Source: CAD feature listing. Evaluate the final solid. Frame: model axes, mm. A direction names the side the tool comes from. Give positions to 0.01 mm unless a question says otherwise; leave off trailing zeros. Order: outer loops, then holes, each group sorted by start corner. A loop starts at its lowest first (then second) coordinate and runs counter-clockwise, first axis right, second up. Notation, with made-up numbers: (68, -28) - (120, -28) arc R23 cw to (120, -15) - close; hole circle Ø7 at (74, 89). An arc over 180 degrees is marked (long way). Write each question's results on one line, items separated by ' | '. Start each with the question number.
Item 1: Line query: line 1 along Y through (x, z) = (9, -4.5); line 2 along X through (y, z) = (-5, -1). Output: solid intervals per line, ascending.
Item 2: Section C-C on y = 8. Output: boundary loops of the cut face in (x, z).
Item 3: Set-up query: faces 1 (the cylindrical face through (-16.129, 16.254, 5.059)), 2 (the flat face through (21, -10.5, -14)), 3 (the conical face through (16.37, 16.24, 3.74)). Return all of +Z, -Z, +X, -X, +Y, -Y with unobstructed straight access to the full face (end or side cutting, diameter ignored); none if empty.
Item 4: Mould query, pull axis Y, two halves, no side actions, for faces 4 (the cylindrical face through (-18.192, 18.363, -12.977)), 5 (the flat face through (-19, 0, 6.25)), 6 (the cylindrical face through (20.514, -9.297, -1.891)). Classes: released by +Y, released by -Y, zero draft, split by the parting line, or undercut.
Item 5: Section B-B on z = -8.5. Output: boundary loops of the cut face in (x, y), and give its area (3 significant figures).
Item 6: Contact query for flat-ended pins moving along their axis: pin 1 Ø1 at (x, z) = (21, -18) entering from +Y; pin 2 Ø2 at (x, z) = (-16, -10) entering from -Y; pin 3 Ø1.6 at (x, z) = (20, -12) entering from -Y. Output: stop coordinate, or through.
Item 7: Section A-A on x = -3. Output: boundary loops of the cut face in (y, z), and give its area (3 significant figures).
Item 8: Section D-D on y = -9.5. Output: boundary loops of the cut face in (x, z), and give its area (3 significant figures).
```python
from build123d import *

# Parameters (mm, degrees)
POWER_BUTTON_HOLE_DEPTH = 2


with BuildPart() as part:
    # Case 2: sweep along a path in Sketch1
    with BuildLine(Plane.XY) as case_2_path:
        Line((-10.5, -19.25), (10.5, -19.25))
        ThreePointArc((10.5, -19.25), (16.687184335, -16.687184335), (19.25, -10.5))
        Line((19.25, -10.5), (19.25, 10.5))
        ThreePointArc((19.25, 10.5), (16.687184335, 16.687184335), (10.5, 19.25))
        Line((10.5, 19.25), (-10.5, 19.25))
        ThreePointArc((-10.5, 19.25), (-16.687184335, 16.687184335), (-19.25, 10.5))
        Line((-19.25, 10.5), (-19.25, -10.5))
        ThreePointArc((-19.25, -10.5), (-16.687184335, -16.687184335), (-10.5, -19.25))
    # Sketch4 → Case 2 (sweep)
    with BuildSketch(Plane(origin=(0, 0, 0), x_dir=(1, 0, 0), z_dir=(0, 1, 0))):
        with BuildLine():
            Line((-19.5, 0), (-19.5, -3))
            Line((-19.5, -3), (-19.45, -3))
            Line((-19.45, -3), (-18.55, -3.9))
            Line((-18.55, -3.9), (-18.55, -6.25))
            Line((-18.55, -6.25), (-21.5, -6.25))
            Line((-21.5, -6.25), (-21.5, 32.75))
            Line((-21.5, 32.75), (-19.5, 32.75))
            Line((-19.5, 32.75), (-19.5, 31.616025404))
            ThreePointArc((-19.5, 31.616025404), (-19.566987298, 31.366025404), (-19.75, 31.183012702))
            ThreePointArc((-19.75, 31.183012702), (-20, 30.75), (-19.75, 30.316987298))
            ThreePointArc((-19.75, 30.316987298), (-19.566987298, 30.133974596), (-19.5, 29.883974596))
            Line((-19.5, 29.883974596), (-19.5, 0))
        make_face()
    sweep(path=case_2_path.line)

    # Sketch6 → Power Button Hole (cut)
    with BuildSketch(Plane(origin=(21.5, 0, 0), x_dir=(0, 0, -1), z_dir=(1, 0, 0))):
        with BuildLine():
            Line((23.75, 10.5), (4.75, 10.5))
            ThreePointArc((4.75, 10.5), (1.921572875, 9.328427125), (0.75, 6.5))
            Line((0.75, 6.5), (0.75, -6.5))
            ThreePointArc((0.75, -6.5), (1.921572875, -9.328427125), (4.75, -10.5))
            Line((4.75, -10.5), (23.75, -10.5))
            ThreePointArc((23.75, -10.5), (26.578427125, -9.328427125), (27.75, -6.5))
            Line((27.75, -6.5), (27.75, 6.5))
            ThreePointArc((27.75, 6.5), (26.578427125, 9.328427125), (23.75, 10.5))
        make_face()
    extrude(amount=-POWER_BUTTON_HOLE_DEPTH, mode=Mode.SUBTRACT)


solid = part.part
```
Evaluation:
1) line 1: y = -21.5 to -19.5, 19.5 to 21.5 | line 2: x = -21.5 to -19.5
2) outline: (-21.5, -32.75) - (-19.5, -32.75) - (-19.5, -31.62) arc R0.5 ccw to (-19.75, -31.18) arc R0.5 cw to (-19.75, -30.32) arc R0.5 ccw to (-19.5, -29.88) - (-19.5, 3) - (-19.45, 3) - (-18.55, 3.9) - (-18.55, 6.25) - (-21.5, 6.25) - close; (18.55, 3.9) - (19.45, 3) - (19.5, 3) - (19.5, -1.04) - (21.5, -1.04) - (21.5, 6.25) - (18.55, 6.25) - close; (19.5, -32.75) - (21.5, -32.75) - (21.5, -27.46) - (19.5, -27.46) - (19.5, -29.88) arc R0.5 ccw to (19.75, -30.32) arc R0.5 cw to (19.75, -31.18) arc R0.5 ccw to (19.5, -31.62) - close
3) face 1: +Z, -Z | face 2: +X | face 3: -Z
4) face 4: released by +Y | face 5: zero draft | face 6: undercut
5) outline: (-21.5, -10.5) arc R11 ccw to (-10.5, -21.5) - (10.5, -21.5) arc R11 ccw to (21.5, -10.5) - (19.5, -10.5) arc R9 cw to (10.5, -19.5) - (-10.5, -19.5) arc R9 cw to (-19.5, -10.5) - (-19.5, 10.5) arc R9 cw to (-10.5, 19.5) - (10.5, 19.5) arc R9 cw to (19.5, 10.5) - (21.5, 10.5) arc R11 ccw to (10.5, 21.5) - (-10.5, 21.5) arc R11 ccw to (-21.5, 10.5) - close | area: 252 mm^2
6) pin 1: stops at y = 15.08 | pin 2: stops at y = -20.54 | pin 3: stops at y = -17.23
7) outline: (-21.5, -32.75) - (-19.5, -32.75) - (-19.5, -31.62) arc R0.5 ccw to (-19.75, -31.18) arc R0.5 cw to (-19.75, -30.32) arc R0.5 ccw to (-19.5, -29.88) - (-19.5, 3) - (-19.45, 3) - (-18.55, 3.9) - (-18.55, 6.25) - (-21.5, 6.25) - close; (18.55, 3.9) - (19.45, 3) - (19.5, 3) - (19.5, -29.88) arc R0.5 ccw to (19.75, -30.32) arc R0.5 cw to (19.75, -31.18) arc R0.5 ccw to (19.5, -31.62) - (19.5, -32.75) - (21.5, -32.75) - (21.5, 6.25) - (18.55, 6.25) - close | area: 160 mm^2
8) outline: (-21.5, -32.75) - (-19.5, -32.75) - (-19.5, -31.62) arc R0.5 ccw to (-19.75, -31.18) arc R0.5 cw to (-19.75, -30.32) arc R0.5 ccw to (-19.5, -29.88) - (-19.5, 3) - (-19.45, 3) - (-18.55, 3.9) - (-18.55, 6.25) - (-21.5, 6.25) - close; (18.55, 3.9) - (19.45, 3) - (19.5, 3) - (19.5, -2.1) - (21.5, -2.1) - (21.5, 6.25) - (18.55, 6.25) - close; (19.5, -32.75) - (21.5, -32.75) - (21.5, -26.4) - (19.5, -26.4) - (19.5, -29.88) arc R0.5 ccw to (19.75, -30.32) arc R0.5 cw to (19.75, -31.18) arc R0.5 ccw to (19.5, -31.62) - close | area: 112 mm^2
